Check sheet for the drawn part. Datum: minimum x, y, z corner. Units: mm. A direction names the side the tool comes from. Coordinates: 2 decimals unless noted, no trailing zeros. Write each loop counter-clockwise with the first axis right and the second up, starting at its lowest first coordinate (ties: lowest second). Pieces come first, ordered by that corner, then holes. Notation, with made-up numbers: (43.5, 34) -> (96.5, 34) arc R11 cw to (96.5, 46) -> close; hole circle Ø8 at (66, -27). An arc over 180 degrees is marked (long way). Answer in a Markdown table with one row per item. Add a question column.
Q1. Thickness scan on line 1 (Y direction, x = 16.5, z = 33); line 2 (X direction, y = 32.5, z = 13.5); line 3 (X direction, y = 21, z = 32). Record the ranges inside material, lowest first.
Q2. Section check D-D, the plane y = 22.5. Record the boundary of the cut face in (x, z), and give its area (3 significant figures).
Q3. Tool access check on the marked faces 1 and 2. Record the directions out of +Z, -Z, +X, -X, +Y, -Y that give a thin tool (end or side, any length) a straight path to the whole face; none if there is none.
Q4. Section check A-A, the plane y = 31.5. Record the boundary of the cut face in (x, z), and give its area (3 significant figures).
Q5. Section check B-B, the plane z = 31.5. Record the boundary of the cut face in (x, y).
Q6. Gauge pin test, flat ends, axial feed: P1, Ø1.5, axis at x = 31.5, z = 21, coming from the +Y side; P2, Ø4, axis at x = 18.5, z = 36.5, coming from the +Y side. Record the tip position at first contact, or that the pin passes through.
Q7. Section check C-C, the plane x = 22. Record the boundary of the cut face in (y, z), and give its area (3 significant figures).
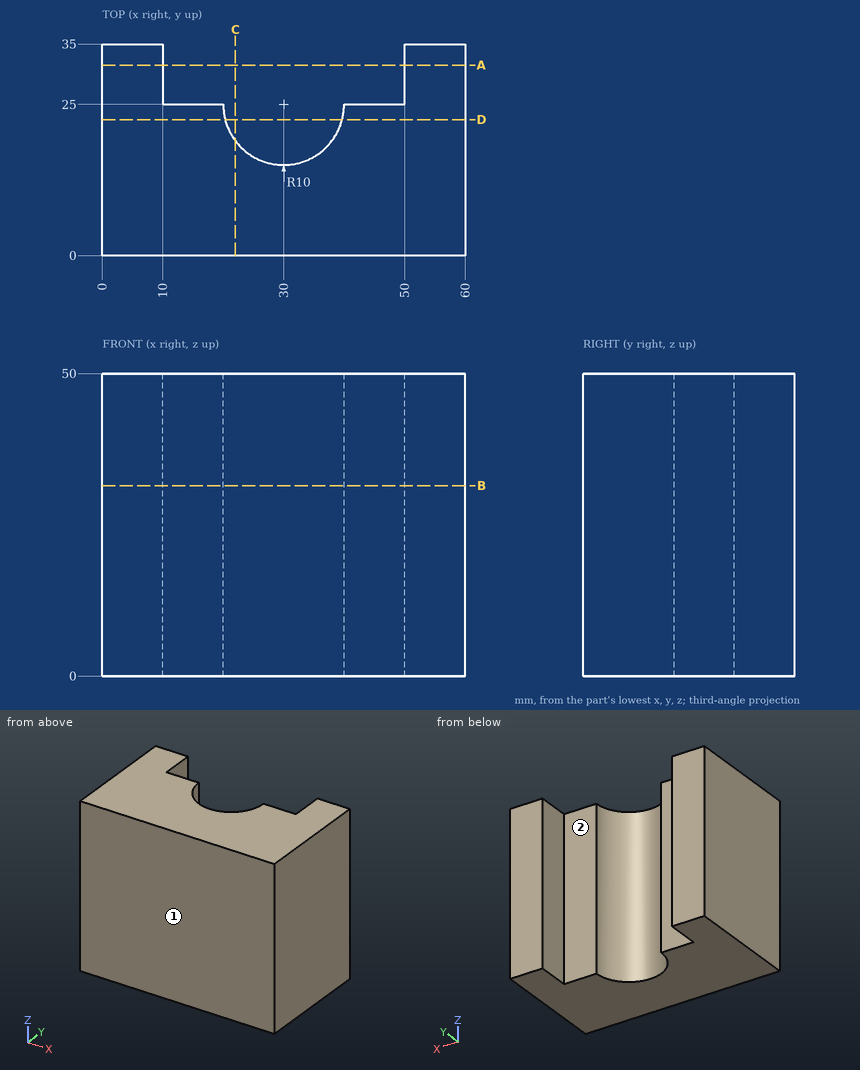
Calculated:
| question | item | result |
|---|---|---|
| 1 | line 1 | y = 0 to 25 |
| 1 | line 2 | x = 0 to 10, 50 to 60 |
| 1 | line 3 | x = 0 to 20.83, 39.17 to 60 |
| 2 | outline | (0, 0) -> (20.32, 0) -> (20.32, 50) -> (0, 50) -> close; (39.68, 0) -> (60, 0) -> (60, 50) -> (39.68, 50) -> close |
| 2 | area | 2,030 mm² |
| 3 | face 1 | +Z, -Z, +X, -X, -Y |
| 3 | face 2 | +Z, -Z, +Y |
| 4 | outline | (0, 0) -> (10, 0) -> (10, 50) -> (0, 50) -> close; (50, 0) -> (60, 0) -> (60, 50) -> (50, 50) -> close |
| 4 | area | 1,000 mm² |
| 5 | outline | (0, 0) -> (60, 0) -> (60, 35) -> (50, 35) -> (50, 25) -> (40, 25) arc R10 cw to (20, 25) -> (10, 25) -> (10, 35) -> (0, 35) -> close |
| 6 | P1 | stops at y = 15.26 |
| 6 | P2 | stops at y = 25 |
| 7 | outline | (0, 0) -> (19, 0) -> (19, 50) -> (0, 50) -> close |
| 7 | area | 950 mm² |
